from build123d import *

# Parameters (mm, degrees)
BOSS_EXTRUDE1_DEPTH              = 1.68939972
F_2_9_2_9_DIAMETER_HOLE1_D       = 2.89999928
F_2_9_2_9_DIAMETER_HOLE1_DEPTH   = 1.68939972
HOLE1_D                          = 1.1999976
HOLE1_DEPTH                      = 1.68939972
LPATTERN1_COUNT                  = 2
LPATTERN1_PITCH                  = 2.540004919
HOLE2_D                          = 0.999998
HOLE2_DEPTH                      = 1.68939972
LPATTERN2_COUNT                  = 2
LPATTERN2_PITCH                  = 2.54
LPATTERN2_COUNT_DIR2             = 10
LPATTERN2_PITCH_DIR2             = 2.54
HOLE3_D                          = 1.1999976
HOLE3_DEPTH                      = 1.68939972
LPATTERN3_COUNT                  = 5
LPATTERN3_PITCH                  = 2.54
F_2_9_2_9_DIAMETER_HOLE2_D       = 2.89999928
F_2_9_2_9_DIAMETER_HOLE2_DEPTH   = 1.68939972
HOLE4_D                          = 1.1999976
HOLE4_DEPTH                      = 1.68939972
LPATTERN4_COUNT                  = 2
LPATTERN4_PITCH                  = 2.540004919
F_0_85_0_85_DIAMETER_HOLE1_D     = 0.85000084
F_0_85_0_85_DIAMETER_HOLE1_DEPTH = 1.68939972
HOLE5_D                          = 0.7999984
HOLE5_DEPTH                      = 1.68939972
LPATTERN5_COUNT                  = 3
LPATTERN5_PITCH                  = 3.99999962
LPATTERN5_COUNT_DIR2             = 2
LPATTERN5_PITCH_DIR2             = 2.50000008
F_2_9_2_9_DIAMETER_HOLE3_D       = 2.89999928
F_2_9_2_9_DIAMETER_HOLE3_DEPTH   = 1.68939972
F_2_9_2_9_DIAMETER_HOLE4_D       = 2.89999928
F_2_9_2_9_DIAMETER_HOLE4_DEPTH   = 1.68939972
F_0_85_0_85_DIAMETER_HOLE2_D     = 0.85000084
F_0_85_0_85_DIAMETER_HOLE2_DEPTH = 1.68939972
HOLE6_D                          = 1.1999976
HOLE6_DEPTH                      = 1.68939972
LPATTERN6_COUNT                  = 2
LPATTERN6_PITCH                  = 12.200001
F_2_9_2_9_DIAMETER_HOLE5_D       = 2.89999928
F_2_9_2_9_DIAMETER_HOLE5_DEPTH   = 1.68939972


with BuildPart() as part:
    # Sketch1 → Boss-Extrude1 (new body)
    with BuildSketch(Plane.XY.offset(1.68939972)):
        with BuildLine():
            Line((87.300003052, 25.399999619), (87.300003052, 29.399999619))
            ThreePointArc((87.300003052, 29.399999619), (87.592896271, 30.1071064), (88.300003052, 30.399999619))
            Line((88.300003052, 30.399999619), (101.5, 30.399999619))
            ThreePointArc((101.5, 30.399999619), (102.207106781, 30.1071064), (102.5, 29.399999619))
            Line((102.5, 29.399999619), (102.5, 25.399999619))
            Line((102.5, 25.399999619), (124.900001526, 25.399999619))
            Line((124.900001526, 25.399999619), (124.900001526, 99.5))
            Line((124.900001526, 99.5), (33.400001526, 99.5))
            Line((33.400001526, 99.5), (33.400001526, 93.949998856))
            ThreePointArc((33.400001526, 93.949998856), (32.374874701, 91.475123773), (29.899999619, 90.449996948))
            Line((29.899999619, 90.449996948), (25.399999619, 90.449996948))
            Line((25.399999619, 90.449996948), (25.399999619, 34.450000763))
            Line((25.399999619, 34.450000763), (29.899999619, 34.450000763))
            ThreePointArc((29.899999619, 34.450000763), (32.374874701, 33.424873938), (33.400001526, 30.949998856))
            Line((33.400001526, 30.949998856), (33.400001526, 25.399999619))
            Line((33.400001526, 25.399999619), (87.300003052, 25.399999619))
        make_face()
    extrude(amount=-BOSS_EXTRUDE1_DEPTH)

    # 2.9 _2.9_ Diameter Hole1
    with Locations(Plane(origin=(0, 0, 0), x_dir=(-1, 0, 0), z_dir=(0, 0, -1))):
        with Locations((-122.39998888, 62.44998432)):
            Hole(F_2_9_2_9_DIAMETER_HOLE1_D / 2, depth=F_2_9_2_9_DIAMETER_HOLE1_DEPTH)

    # Hole1
    with Locations(Plane(origin=(0, 0, 0), x_dir=(-1, 0, 0), z_dir=(0, 0, -1))):
        with Locations((-107.44449936, 78.74)):
            hole1 = Hole(HOLE1_D / 2, depth=HOLE1_DEPTH)

    # LPattern1: Hole1 ×2
    with Locations(*[Vector(-0.001967996, -0.999998063, 0) * (i * LPATTERN1_PITCH) for i in range(1, LPATTERN1_COUNT)]):
        add(hole1, mode=Mode.SUBTRACT)

    # Hole2
    with Locations(Plane(origin=(0, 0, 0), x_dir=(-1, 0, 0), z_dir=(0, 0, -1))):
        with Locations((-113.284, 38.227)):
            hole2 = Hole(HOLE2_D / 2, depth=HOLE2_DEPTH)

    # LPattern2: Hole2 2 × 10
    with Locations(*[(i * LPATTERN2_PITCH, j * LPATTERN2_PITCH_DIR2, 0) for i in range(LPATTERN2_COUNT) for j in range(LPATTERN2_COUNT_DIR2) if (i, j) != (0, 0)]):
        add(hole2, mode=Mode.SUBTRACT)

    # Hole3
    with Locations(Plane(origin=(0, 0, 0), x_dir=(-1, 0, 0), z_dir=(0, 0, -1))):
        with Locations((-107.442, 94.361)):
            hole3 = Hole(HOLE3_D / 2, depth=HOLE3_DEPTH)

    # LPattern3: Hole3 ×5
    with Locations(*[(0, -i * LPATTERN3_PITCH, 0) for i in range(1, LPATTERN3_COUNT)]):
        add(hole3, mode=Mode.SUBTRACT)

    # 2.9 _2.9_ Diameter Hole2
    with Locations(Plane(origin=(0, 0, 0), x_dir=(-1, 0, 0), z_dir=(0, 0, -1))):
        with Locations((-33.399984, 84.94998504)):
            Hole(F_2_9_2_9_DIAMETER_HOLE2_D / 2, depth=F_2_9_2_9_DIAMETER_HOLE2_DEPTH)

    # Hole4
    with Locations(Plane(origin=(0, 0, 0), x_dir=(-1, 0, 0), z_dir=(0, 0, -1))):
        with Locations((-107.43950064, 68.326)):
            hole4 = Hole(HOLE4_D / 2, depth=HOLE4_DEPTH)

    # LPattern4: Hole4 ×2
    with Locations(*[Vector(0.001967996, 0.999998063, 0) * (i * LPATTERN4_PITCH) for i in range(1, LPATTERN4_COUNT)]):
        add(hole4, mode=Mode.SUBTRACT)

    # 0.85 _0.85_ Diameter Hole1
    with Locations(Plane(origin=(0, 0, 0), x_dir=(-1, 0, 0), z_dir=(0, 0, -1))):
        with Locations((-27.25008266, 65.84998768)):
            Hole(F_0_85_0_85_DIAMETER_HOLE1_D / 2, depth=F_0_85_0_85_DIAMETER_HOLE1_DEPTH)

    # Hole5
    with Locations(Plane(origin=(0, 0, 0), x_dir=(-1, 0, 0), z_dir=(0, 0, -1))):
        with Locations((-90.29998196, 36.04998632)):
            hole5 = Hole(HOLE5_D / 2, depth=HOLE5_DEPTH)

    # LPattern5: Hole5 3 × 2
    with Locations(*[(i * LPATTERN5_PITCH, -j * LPATTERN5_PITCH_DIR2, 0) for i in range(LPATTERN5_COUNT) for j in range(LPATTERN5_COUNT_DIR2) if (i, j) != (0, 0)]):
        add(hole5, mode=Mode.SUBTRACT)

    # 2.9 _2.9_ Diameter Hole3
    with Locations(Plane(origin=(0, 0, 0), x_dir=(-1, 0, 0), z_dir=(0, 0, -1))):
        with Locations((-33.399984, 39.9499836)):
            Hole(F_2_9_2_9_DIAMETER_HOLE3_D / 2, depth=F_2_9_2_9_DIAMETER_HOLE3_DEPTH)

    # 2.9 _2.9_ Diameter Hole4
    with Locations(Plane(origin=(0, 0, 0), x_dir=(-1, 0, 0), z_dir=(0, 0, -1))):
        with Locations((-46.1999838, 34.44998952)):
            Hole(F_2_9_2_9_DIAMETER_HOLE4_D / 2, depth=F_2_9_2_9_DIAMETER_HOLE4_DEPTH)

    # 0.85 _0.85_ Diameter Hole2
    with Locations(Plane(origin=(0, 0, 0), x_dir=(-1, 0, 0), z_dir=(0, 0, -1))):
        with Locations((-27.25008266, 59.04998604)):
            Hole(F_0_85_0_85_DIAMETER_HOLE2_D / 2, depth=F_0_85_0_85_DIAMETER_HOLE2_DEPTH)

    # Hole6
    with Locations(Plane(origin=(0, 0, 0), x_dir=(-1, 0, 0), z_dir=(0, 0, -1))):
        with Locations((-88.19998108, 34.79998628)):
            hole6 = Hole(HOLE6_D / 2, depth=HOLE6_DEPTH)

    # LPattern6: Hole6 ×2
    with Locations(*[(i * LPATTERN6_PITCH, 0, 0) for i in range(1, LPATTERN6_COUNT)]):
        add(hole6, mode=Mode.SUBTRACT)

    # 2.9 _2.9_ Diameter Hole5
    with Locations(Plane(origin=(0, 0, 0), x_dir=(-1, 0, 0), z_dir=(0, 0, -1))):
        with Locations((-46.1999838, 90.44998928)):
            Hole(F_2_9_2_9_DIAMETER_HOLE5_D / 2, depth=F_2_9_2_9_DIAMETER_HOLE5_DEPTH)


solid = part.part
Source: CAD feature listing. Evaluate the final solid. Frame: model axes, mm. Round coordinates to 2 decimals unless told otherwise and drop trailing zeros. Use a Markdown table: item, result. Add a question column.
1. First-contact query: pin 1 (0.8 mm diameter, centred on y = 29.5, z = 0.5, fed in from -X); pin 2 (0.8 mm diameter, centred on x = 28, z = 1, fed in from +Y). Flat tips, straight axial feed; report the tip coordinate or a pass-through.
2. Section query A-A (z = 0.7). Give the number of separate pieces and of enclosed holes in the cut face, then the cut area to 3 significant figures.
3. Line query: probe 1 along X at (y, z) = (56, 0.3); probe 2 along Y at (x, z) = (33.5, 1.45); probe 3 along X at (y, z) = (43, 1). Output: solid intervals per line, ascending.
4. Mould query, pull axis X, two halves, no side actions, for faces 1 (the cylindrical face through (122.086, 61.034, 0.857)), 2 (the cylindrical face through (32.3, 33.5, 0.9)), 3 (the flat face through (74, 63, 0)). Classes: +X half, -X half, draft (parallel to the pull), parting line (faces both ways), or undercut.
Derived:
| question | item | result |
|---|---|---|
| 1 | pin 1 | x = 33.4 |
| 1 | pin 2 | y = 90.45 |
| 2 | separate pieces | 1 |
| 2 | enclosed holes | 44 |
| 2 | area | 7,090 mm2 |
| 3 | probe 1 | 25.4 to 112.78, 113.78 to 115.32, 116.32 to 124.9 |
| 3 | probe 2 | 25.4 to 38.5, 41.4 to 83.5, 86.4 to 99.5 |
| 3 | probe 3 | 25.4 to 112.89, 113.68 to 115.43, 116.22 to 124.9 |
| 4 | face 1 | undercut |
| 4 | face 2 | -X half |
| 4 | face 3 | draft |
